Geometry: see drawing. Coordinates: mm, zero at the bounding-box minimum. Round coordinates to 2 decimals unless told otherwise and drop trailing zeros. Write each loop counter-clockwise with the first axis right and the second up, starting at its lowest first coordinate (ties: lowest second). Pieces come first, ordered by that corner, then holes. Notation, with made-up numbers: M 21.5,-21 L 38.5,-21 A19 ccw 38.5,4 Z; hole C 49,22 d3. An arc over 180 degrees is marked long. Use one line per item in the form item = value. Start each with the question number.
Item 1: Section query B-B (z = 16.5). Return loops of the section in (x, y).
Item 2: Section query A-A (y = 1.5). Return loops of the section in (x, z).
Item 3: Pin query (flat end, axial travel): pin 1 Ø1.5 at (x, y) = (39.5, 1.5) entering from +Z; pin 2 Ø1.5 at (y, z) = (2, 3.5) entering from -X; pin 3 Ø0.9 at (y, z) = (2, 32) entering from +X. Return the tip coordinate at first contact, or that it passes through.
Item 4: Ray query, probe 1 along Z at (x, y) = (39.5, 1.7); probe 2 along X at (y, z) = (2.15, 2). Return the intervals inside material, ascending.
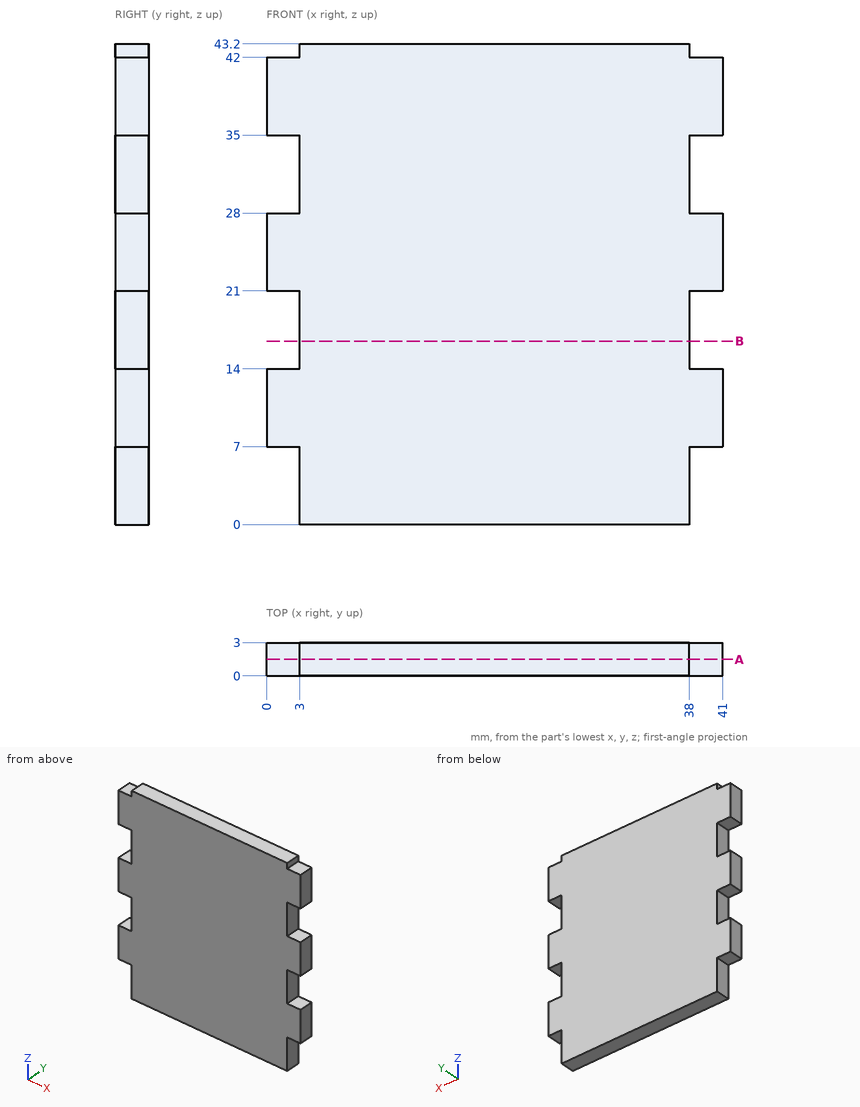
Working result:
q1.outline = M 3,0 L 38,0 L 38,3 L 3,3 Z
q2.outline = M 0,7 L 3,7 L 3,0 L 38,0 L 38,7 L 41,7 L 41,14 L 38,14 L 38,21 L 41,21 L 41,28 L 38,28 L 38,35 L 41,35 L 41,42 L 38,42 L 38,43.2 L 3,43.2 L 3,42 L 0,42 L 0,35 L 3,35 L 3,28 L 0,28 L 0,21 L 3,21 L 3,14 L 0,14 Z
q3.pin_1 = 42
q3.pin_2 = 3
q3.pin_3 = 38
q4.probe_1 = 7 to 14, 21 to 28, 35 to 42
q4.probe_2 = 3 to 38
